```python
from build123d import *

# Parameters (mm, degrees)
SKETCH1_R           = 3.96875
BOSS_EXTRUDE1_DEPTH = 9.525


with BuildPart() as part:
    # Sketch1 → Boss-Extrude1 (new, symmetric)
    with BuildSketch(Plane.XY):
        with BuildLine():
            Line((-63.5, -25.4), (63.5, -25.4))
            ThreePointArc((63.5, -25.4), (88.9, 0), (63.5, 25.4))
            Line((63.5, 25.4), (-63.5, 25.4))
            ThreePointArc((-63.5, 25.4), (-88.9, 0), (-63.5, -25.4))
        make_face()
        with Locations(Location((-69.85, 0, 0), (0, 0, 180))):
            Circle(SKETCH1_R, mode=Mode.SUBTRACT)
        with Locations(Location((69.85, 0, 0), (0, 0, 180))):
            Circle(SKETCH1_R, mode=Mode.SUBTRACT)
    extrude(amount=BOSS_EXTRUDE1_DEPTH, both=True)


solid = part.part
```
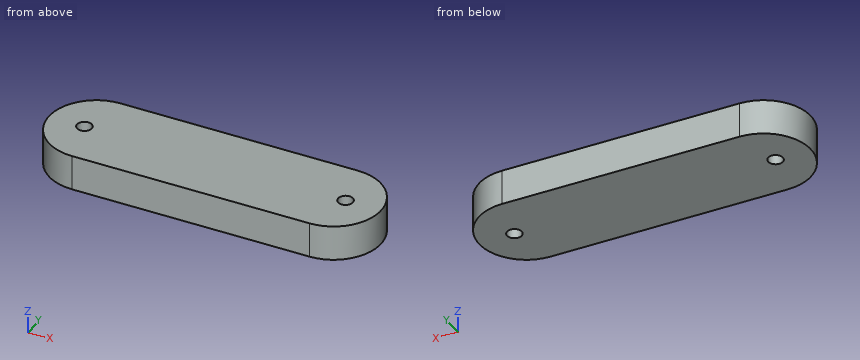
CAD build for the part. Positions are in the model's coordinates, mm. Round coordinates to 2 decimals unless told otherwise and drop trailing zeros. Write each loop counter-clockwise with the first axis right and the second up, starting at its lowest first coordinate (ties: lowest second). Pieces come first, ordered by that corner, then holes. Notation, with made-up numbers: (61.5, -25) - (73.5, -25) arc R22 ccw to (73.5, -19) - close; hole circle Ø4 at (-20.75, -2.5). An arc over 180 degrees is marked (long way). Write item = value, one per line. Start each with the question number.
Q1. Probe L1, parallel to X at y = -3.5, z = -2.5; L2, parallel to Y at x = -69.85, z = 4; L3, parallel to X at y = -3, z = 7.75. List the from-to ranges inside material, lowest first. Write a range as from..to.
Q2. Band-saw the part on C-C (z = -7). Give the cut face in (x, y).
Q3. Band-saw the part on A-A (y = 0). Give the cut face in (x, z) (3 decimals).
Q4. Band-saw the part on B-B (x = 69.85). Give the cut face in (y, z) (3 decimals), then the cut area to 3 significant figures.
Q5. Drop flat-ended pins along their axis: pin 1 (10 mm diameter, centred on x = 70.5, z = 6, fed in from +Y); pin 2 (1.5 mm diameter, centred on x = 70.5, z = -3.5, fed in from -Y). Give the stop position or say it passes through.
Q6. Band-saw the part on D-D (x = -75.5). Give the cut face in (y, z) (3 decimals).
Answers below:
q1.L1 = -88.66..-71.72, -67.98..67.98, 71.72..88.66
q1.L2 = -24.59..-3.97, 3.97..24.59
q1.L3 = -88.72..-72.45, -67.25..67.25, 72.45..88.72
q2.outline = (-63.5, -25.4) - (63.5, -25.4) arc R25.4 ccw to (63.5, 25.4) - (-63.5, 25.4) arc R25.4 ccw to start; hole circle Ø7.94 at (-69.85, 0); hole circle Ø7.94 at (69.85, 0)
q3.outline = (-88.9, -9.525) - (-73.819, -9.525) - (-73.819, 9.525) - (-88.9, 9.525) - close; (-65.881, -9.525) - (65.881, -9.525) - (65.881, 9.525) - (-65.881, 9.525) - close; (73.819, -9.525) - (88.9, -9.525) - (88.9, 9.525) - (73.819, 9.525) - close
q4.outline = (-24.593, -9.525) - (-3.969, -9.525) - (-3.969, 9.525) - (-24.593, 9.525) - close; (3.969, -9.525) - (24.593, -9.525) - (24.593, 9.525) - (3.969, 9.525) - close
q4.area = 786 mm2
q5.pin_1 = 25.32
q5.pin_2 = -24.62
q6.outline = (-22.387, -9.525) - (22.387, -9.525) - (22.387, 9.525) - (-22.387, 9.525) - close
